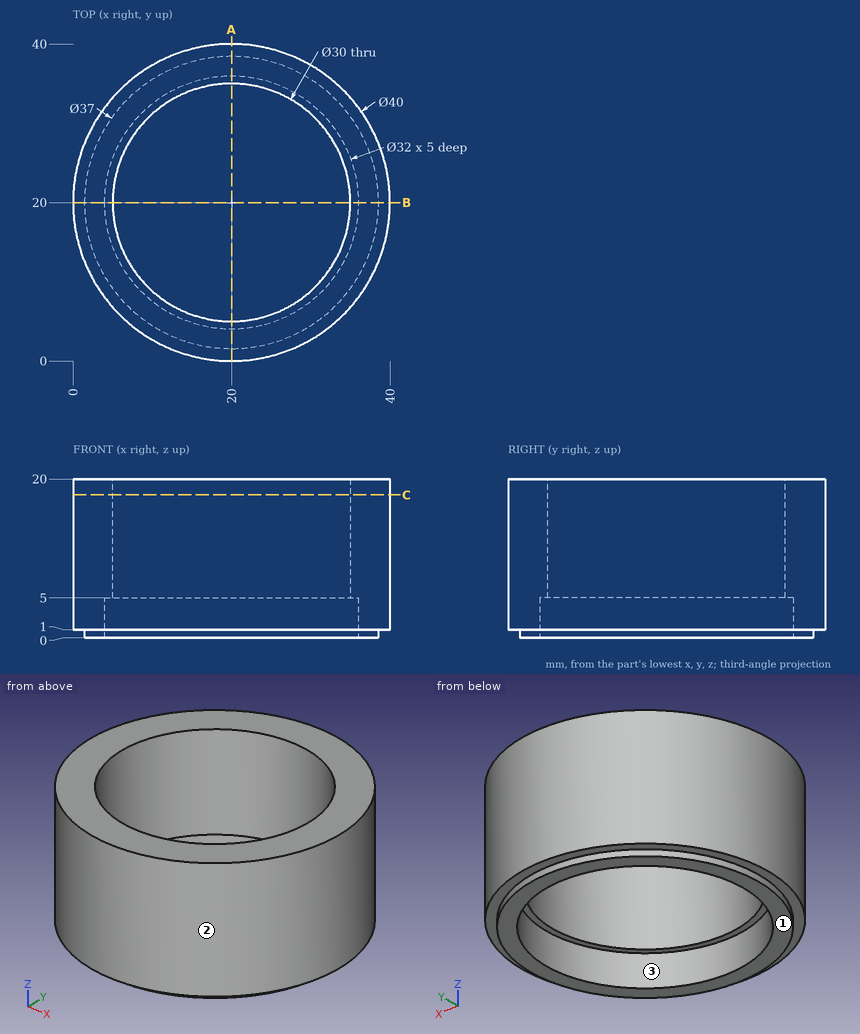
Drawing for the job (mm, zero at the part's lowest x, y, z). Round coordinates to 2 decimals unless told otherwise and drop trailing zeros. Write each loop counter-clockwise with the first axis right and the second up, starting at its lowest first coordinate (ties: lowest second). Pieces come first, ordered by that corner, then holes. Notation, with made-up numbers: (-12, -31.5) - (8, -31.5) arc R18 cw to (8, -20.5) - close; hole circle Ø5 at (29, -22). An arc over 180 degrees is marked (long way). Write item = value, one per line. Start each with the question number.
Q1. Band-saw the part on C-C (z = 18). Give the cut face in (x, y), then the cut area to 3 significant figures.
Q2. Band-saw the part on A-A (x = 20). Give the cut face in (y, z).
Q3. Drop flat-ended pins along their axis: pin 1 (19 mm diameter, centred on x = 20, y = 20, fed in from -Z); pin 2 (8 mm diameter, centred on y = 36, z = 8, fed in from +X); pin 3 (10 mm diameter, centred on x = 6, z = 11, fed in from +Y); pin 4 (1 mm diameter, centred on x = 32, z = 11.5, fed in from +Y). Give the stop position or say it passes through.
Q4. Mould opens along Y. For the marked faces 1, 2 and 3 say: pulls with the +Y half, pulls with the -Y half, needs draft (parallel to the pull), parting line crosses it, or undercut.
Q5. Probe L1, parallel to Y at x = 20, z = 3.8; L2, parallel to Y at x = 20, z = 14.5; L3, parallel to X at y = 25, z = 3.5. List the from-to ranges inside material, lowest first. Write a range as from..to.
Answers below:
q1.outline = circle Ø40 at (20, 20); hole circle Ø30 at (20, 20)
q1.area = 550 mm2
q2.outline = (0, 1) - (1.5, 1) - (1.5, 0) - (4, 0) - (4, 5) - (5, 5) - (5, 20) - (0, 20) - close; (35, 5) - (36, 5) - (36, 0) - (38.5, 0) - (38.5, 1) - (40, 1) - (40, 20) - (35, 20) - close
q3.pin_1 = through
q3.pin_2 = 36
q3.pin_3 = 37.86
q3.pin_4 = 36.36
q4.face_1 = needs draft
q4.face_2 = parting line crosses it
q4.face_3 = undercut
q5.L1 = 0..4, 36..40
q5.L2 = 0..5, 35..40
q5.L3 = 0.64..4.8, 35.2..39.36
